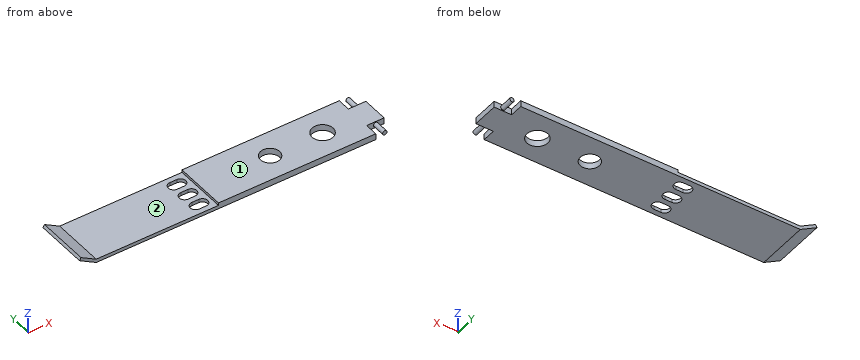
from build123d import *

# Parameters (mm, degrees)
F1_DEPTH  = 30
F2_W      = 15
F2_H      = 3.5
F3_DEPTH  = 10
F4_R      = 1.25
F5_DEPTH  = 7.5
F6_R      = 1.25
F7_DEPTH  = 7.5
F9_DEPTH  = 25
F10_R     = 6
F10_R_2   = 5.5
F11_DEPTH = 25


with BuildPart() as f1:
    # F0 (on Front) → F1 (new body)
    with BuildSketch(Plane.XZ):
        Polygon((-8.73931, 2), (-78.73931, 2), (-87.399564, 7), (-88.265589, 5.5), (-78.73931, 0), (-8.73931, 0), (81.26069, 0), (81.26069, 3.5), (-8.73931, 3.5), align=None)
    extrude(amount=F1_DEPTH)

    # F2 (on face) → F3 (join)
    with BuildSketch(Plane.YZ.offset(81.26069)):
        with Locations((-15, 1.75)):
            Rectangle(F2_W, F2_H)
    extrude(amount=F3_DEPTH)

    # F4 (on face) → F5 (join)
    with BuildSketch(Plane.XZ.offset(22.5)):
        with Locations((86.425211, 1.75)):
            Circle(F4_R)
    extrude(amount=F5_DEPTH)

    # F6 (on face) → F7 (join)
    with BuildSketch(Plane(origin=(0, -7.5, 0), x_dir=(-1, 0, 0), z_dir=(0, 1, 0))):
        with Locations((-86.26069, 1.75)):
            Circle(F6_R)
    extrude(amount=F7_DEPTH)

    # F8 (on face) → F9 (cut)
    with BuildSketch(Plane.XY.offset(2)):
        with BuildLine():
            Line((-17.73931, -18), (-13.73931, -18))
            ThreePointArc((-13.73931, -18), (-10.73931, -15), (-13.73931, -12))
            Line((-13.73931, -12), (-17.73931, -12))
            ThreePointArc((-17.73931, -12), (-20.73931, -15), (-17.73931, -18))
        make_face()
        with BuildLine():
            Line((-13.73931, -21), (-17.73931, -21))
            ThreePointArc((-17.73931, -21), (-20.73931, -24), (-17.73931, -27))
            Line((-17.73931, -27), (-13.73931, -27))
            ThreePointArc((-13.73931, -27), (-10.73931, -24), (-13.73931, -21))
        make_face()
        with BuildLine():
            ThreePointArc((-17.73931, -3), (-20.73931, -6), (-17.73931, -9))
            Line((-17.73931, -9), (-13.73931, -9))
            ThreePointArc((-13.73931, -9), (-10.73931, -6), (-13.73931, -3))
            Line((-13.73931, -3), (-17.73931, -3))
        make_face()
    extrude(amount=-F9_DEPTH, mode=Mode.SUBTRACT)

    # F10 (on face) → F11 (cut)
    with BuildSketch(Plane.XY.offset(3.5)):
        with Locations((61.26069, -15)):
            Circle(F10_R)
        with Locations((31.26069, -15)):
            Circle(F10_R_2)
    extrude(amount=-F11_DEPTH, mode=Mode.SUBTRACT)


solid = f1.part
Check sheet for the modelled part. Datum: model origin and axes. Units: mm. Face numbers are marked on the shaded views. Coordinates: 2 decimals unless noted, no trailing zeros. Loops run counter-clockwise (first coordinate to the right, second up) from the corner with the lowest first, then second, coordinate; pieces in that order, holes last. Notation, with made-up numbers: (49.5, -39) -> (93.5, -39) arc R20 ccw to (93.5, -27) -> close; hole circle Ø3 at (67, 8.25). An arc over 180 degrees is marked (long way). Write item = value, one per line. Start each with the question number.
1. Section check A-A on y = -6. Record the cut outline in (x, z).
2. Material ranges on line 1 (Z direction, x = -28, y = -8.25); line 2 (X direction, y = -10.75, z = 2.5); line 3 (Z direction, x = 61, y = -5), recorded low to high.
3. Section check C-C on x = 61.5. Record the cut outline in (y, z).
4. Section check B-B on y = -15. Record the cut outline in (x, z).
5. Depth check by flat-ended pin: P1, Ø6, axis at x = -44.5, y = -18, coming from the +Z side; P2, Ø0.8, axis at y = -19.5, z = 2.5, coming from the -X side; P3, Ø3, axis at y = -25.5, z = 2.5, coming from the +X side. Enter the tip coordinate at first touch or a pass-through.
6. Draft check along X on the marked faces 1 and 2. Enter one of: released by +X, released by -X, zero draft, split by the parting line, or undercut.
7. Section check D-D on x = -50.5. Record the cut outline in (y, z), then the cut area to 3 significant figures.
Responses:
q1.outline = (-88.27, 5.5) -> (-78.74, 0) -> (-20.74, 0) -> (-20.74, 2) -> (-78.74, 2) -> (-87.4, 7) -> close; (-10.74, 0) -> (81.26, 0) -> (81.26, 3.5) -> (-8.74, 3.5) -> (-8.74, 2) -> (-10.74, 2) -> close; circle Ø2.5 at (86.26, 1.75)
q2.line_1 = 0 to 2
q2.line_2 = -83.07 to -79.61, -8.74 to 27.77, 34.75 to 57.03, 65.5 to 91.26
q2.line_3 = 0 to 3.5
q3.outline = (-30, 0) -> (-21, 0) -> (-21, 3.5) -> (-30, 3.5) -> close; (-9, 0) -> (0, 0) -> (0, 3.5) -> (-9, 3.5) -> close
q4.outline = (-88.27, 5.5) -> (-78.74, 0) -> (-20.74, 0) -> (-20.74, 2) -> (-78.74, 2) -> (-87.4, 7) -> close; (-10.74, 0) -> (25.76, 0) -> (25.76, 3.5) -> (-8.74, 3.5) -> (-8.74, 2) -> (-10.74, 2) -> close; (36.76, 0) -> (55.26, 0) -> (55.26, 3.5) -> (36.76, 3.5) -> close; (67.26, 0) -> (91.26, 0) -> (91.26, 3.5) -> (67.26, 3.5) -> close
q5.P1 = 2
q5.P2 = -83.76
q5.P3 = 87.68
q6.face_1 = zero draft
q6.face_2 = undercut
q7.outline = (-30, 0) -> (0, 0) -> (0, 2) -> (-30, 2) -> close
q7.area = 60.0 mm2
